Could you check a few things on this drawing? It's one solid part, dimensions in mm from its lowest x, y, z. A direction names the side the tool comes from. Round coordinates to 2 decimals unless told otherwise and drop trailing zeros. Loops run counter-clockwise (first coordinate to the right, second up) from the corner with the lowest first, then second, coordinate; pieces in that order, holes last. Notation, with made-up numbers: M 13,26 L 49,26 A8 cw 49,39 Z; hole C 22,-2.5 d10. An arc over 180 degrees is marked long. Use a Markdown table: item, result. Add a question column.
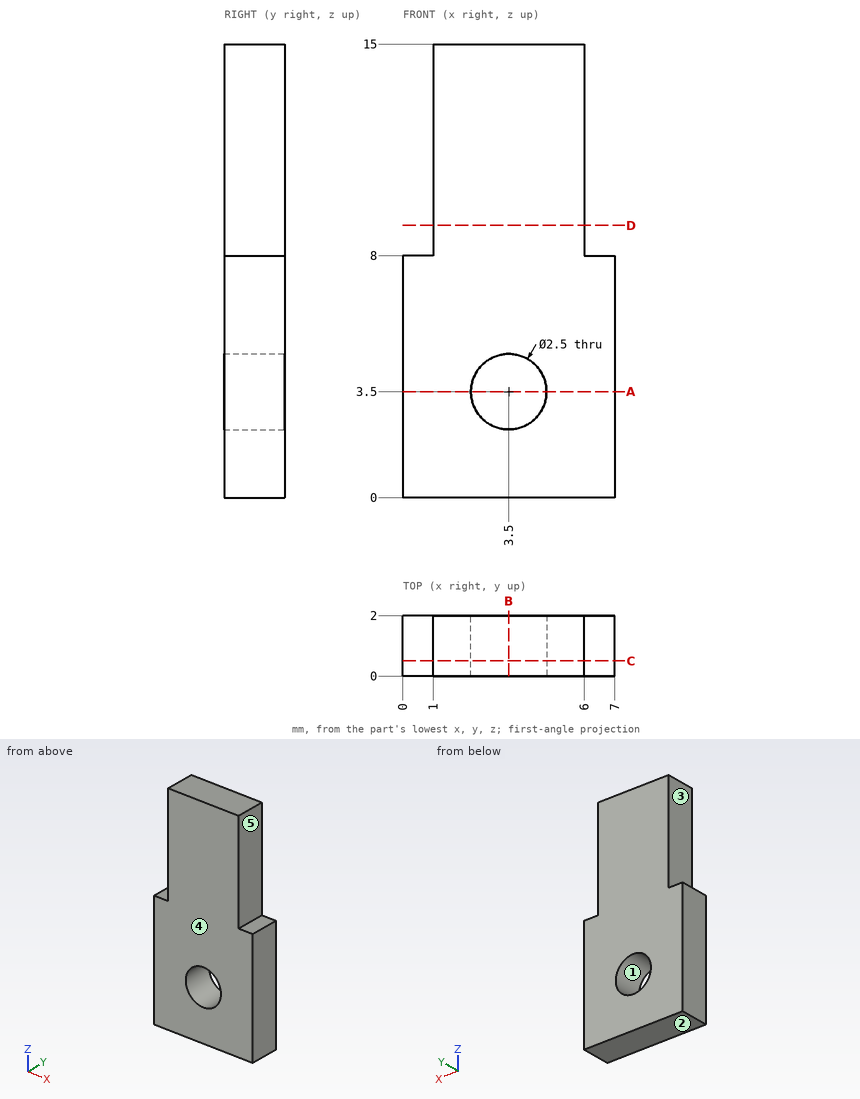
(1) Thinking about a two-plate mould opening in Z: for the marked faces 1, 2 and 3, which applies, released by +Z, released by -Z, zero draft, split by the parting line, or undercut?
(2) Suppose I cut it at D-D on z = 9. List the corners of the cut face in (x, y) for me.
(3) I'm going to push a flat-ended pin straight in: pin 1 (0.8 mm diameter, centred on x = 6.5, y = 0.5, fed in from +Z). Where does the tip first touch, or does it pass through?
(4) If I drill on probe 1 along X at (y, z) = (0.45, 3.5); probe 2 along Z at (x, y) = (3.5, 0.8); probe 3 along X at (y, z) = (0.1, 13), over which ranges is the centre line in solid material (lowest first)? Write a range as [from, to].
(5) Suppose I cut it at B-B on x = 3.5. List the corners of the cut face in (y, z) for me.
(6) On a 3-axis mill with a long thin cutter (end or side, diameter ignored), from which of +Z, -Z, +X, -X, +Y, -Y can I reach the whole of each face in a straight line? I mean the marked faces 4 and 5. Say none if no direction works.
(7) Suppose I cut it at C-C on y = 0.5. List the corners of the cut face in (x, z) for me, and give its area (3 significant figures).
(8) Suppose I cut it at A-A on z = 3.5. List the corners of the cut face in (x, y) for me.
Results below:
| question | item | result |
|---|---|---|
| 1 | face 1 | undercut |
| 1 | face 2 | released by -Z |
| 1 | face 3 | zero draft |
| 2 | outline | M 1,0 L 6,0 L 6,2 L 1,2 Z |
| 3 | pin 1 | stops at z = 8 |
| 4 | probe 1 | x = [0, 2.25], [4.75, 7] |
| 4 | probe 2 | z = [0, 2.25], [4.75, 15] |
| 4 | probe 3 | x = [1, 6] |
| 5 | outline | M 0,0 L 2,0 L 2,2.25 L 0,2.25 Z; M 0,4.75 L 2,4.75 L 2,15 L 0,15 Z |
| 6 | face 4 | +Z, -Z, +X, -X, -Y |
| 6 | face 5 | +Z, +X, +Y, -Y |
| 7 | outline | M 0,0 L 7,0 L 7,8 L 6,8 L 6,15 L 1,15 L 1,8 L 0,8 Z; hole C 3.5,3.5 d2.5 |
| 7 | area | 86.1 mm² |
| 8 | outline | M 0,0 L 2.25,0 L 2.25,2 L 0,2 Z; M 4.75,0 L 7,0 L 7,2 L 4.75,2 Z |
